Geometry check sheet. Reference: the model listing, model coordinates, mm. A direction names the side the tool comes from. Coordinates: 2 decimals unless noted, no trailing zeros. Write each loop counter-clockwise with the first axis right and the second up, starting at its lowest first coordinate (ties: lowest second). Pieces come first, ordered by that corner, then holes. Notation, with made-up numbers: (67.25, 61.25) -> (104.25, 61.25) arc R23 cw to (104.25, 99.25) -> close; hole circle Ø6 at (24.5, 37). An arc over 180 degrees is marked (long way). One line per question, with ' | ' between items.
from build123d import *

# Parameters (mm, degrees)
SKETCH_1_W          = 10
SKETCH_1_H          = 335
SKETCH_1_R          = 1.6
EXTRUDE_1_DEPTH     = 10
SKETCH_2_W          = 8
SKETCH_2_H          = 8
CUT_EXTRUDE_1_DEPTH = 1000


with BuildPart() as part:
    # ｽｹｯﾁ1 → ﾎﾞｽ - 押し出し1 (new body)
    with BuildSketch(Plane.XY):
        with Locations((5, 167.5)):
            Rectangle(SKETCH_1_W, SKETCH_1_H)
        with Locations((5, 326.683332908)):
            Circle(SKETCH_1_R, mode=Mode.SUBTRACT)
        with Locations((5, 7.5)):
            Circle(SKETCH_1_R, mode=Mode.SUBTRACT)
    extrude(amount=EXTRUDE_1_DEPTH)

    # ｽｹｯﾁ2 → ｶｯﾄ - 押し出し1 (cut)
    with BuildSketch(Plane.XZ):
        with Locations((5, 5)):
            Rectangle(SKETCH_2_W, SKETCH_2_H)
    extrude(amount=-CUT_EXTRUDE_1_DEPTH, mode=Mode.SUBTRACT)


solid = part.part
1. Mould release check, pull along Z, two halves, no side actions. Record for faces 1 (the face through (9, 165, 5)), 2 (the face through (5, 170, 10)), 3 (the face through (4.9, 0, 9.4)): released by +Z, released by -Z, zero draft, split by the parting line, or undercut.
Worked answers:
face 1: undercut | face 2: released by +Z | face 3: zero draft
2. Cross-section at B-B on z = 2.75. Record the boundary of the cut face in (x, y).
Worked answers:
outline: (0, 0) -> (1, 0) -> (1, 335) -> (0, 335) -> close; (9, 0) -> (10, 0) -> (10, 335) -> (9, 335) -> close
3. Material ranges on line 1 (Y direction, x = 5, z = 0.55); line 2 (Z direction, x = 5.5, y = 95); line 3 (X direction, y = 7.5, z = 9.5), recorded low to high. Write a range as from..to.
Worked answers:
line 1: 0..5.9, 9.1..325.08, 328.28..335 | line 2: 0..1, 9..10 | line 3: 0..3.4, 6.6..10
4. Cross-section at C-C on x = 5. Record the boundary of the cut face in (y, z), and give its area (3 significant figures).
Worked answers:
outline: (0, 0) -> (5.9, 0) -> (5.9, 1) -> (0, 1) -> close; (0, 9) -> (5.9, 9) -> (5.9, 10) -> (0, 10) -> close; (9.1, 0) -> (325.08, 0) -> (325.08, 1) -> (9.1, 1) -> close; (9.1, 9) -> (325.08, 9) -> (325.08, 10) -> (9.1, 10) -> close; (328.28, 0) -> (335, 0) -> (335, 1) -> (328.28, 1) -> close; (328.28, 9) -> (335, 9) -> (335, 10) -> (328.28, 10) -> close | area: 657 mm²
5. Tool access check on faces 4 (the face through (5, 165, 9)), 5 (the face through (5, 170, 0)). Record the directions out of +Z, -Z, +X, -X, +Y, -Y that give a thin tool (end or side, any length) a straight path to the whole face; none if there is none.
Worked answers:
face 4: +Y, -Y | face 5: -Z, +X, -X, +Y, -Y
6. Cross-section at A-A on y = 62. Record the boundary of the cut face in (x, z).
Worked answers:
outline: (0, 0) -> (10, 0) -> (10, 10) -> (0, 10) -> close; hole (1, 1) -> (9, 1) -> (9, 9) -> (1, 9) -> close
